Geometry check sheet. Reference: the model listing, model coordinates, mm. Face numbers are marked on the shaded views. A direction names the side the tool comes from. Round coordinates to 2 decimals unless told otherwise and drop trailing zeros. Order: outer loops, then holes, each group sorted by start corner. A loop starts at its lowest first (then second) coordinate and runs counter-clockwise, first axis right, second up.
(1) Cross-section at B-B on x = 26.5. Enter the section's corners in (y, z).
(2) Draft check along X on the marked faces 1, 2, 3 and 4. Enter one of: pulls with the +X half, pulls with the -X half, needs draft (parallel to the pull), parting line crosses it, or undercut.
(3) Gauge pin test, flat ends, axial feed: P1, Ø2, axis at x = 19.5, y = 10.5, coming from the +Z side; P2, Ø13.5, axis at y = 14.5, z = 5, coming from the +X side; P3, Ø3.5, axis at x = -6.5, z = 1.5, coming from the +Y side; P4, Ø11.5, axis at y = 25.5, z = 1, coming from the +X side. Record the tip position at first contact, or that the pin passes through.
(4) Cross-section at A-A on y = 25. Enter the section's corners in (x, z).
(5) Cross-section at D-D on y = 5. Enter the section's corners in (x, z), and give its area (4 significant figures).
(6) Thickness scan on L1, parallel to Z at x = 3.5, y = 7; L2, parallel to X at y = 8, z = 0; L3, parallel to Z at x = 23, y = 30.5. Record the ranges inside material, lowest first.
(7) Set-up check for the marked faces 5, 6 and 7: record each of +Z, -Z, +X, -X, +Y, -Y from which the full face is reachable in a straight line by a thin tool's end or side.
(8) Cross-section at C-C on z = 4.75. Enter the section's corners in (x, y), and give its area (3 significant figures).
from build123d import *

# Parameters (mm, degrees)
SKETCH1_W           = 38
SKETCH1_H           = 20
BOSS_EXTRUDE1_DEPTH = 32
SKETCH2_W           = 35
SKETCH2_H           = 17
CUT_EXTRUDE1_DEPTH  = 28
SKETCH3_W           = 4.5
SKETCH3_H           = 17
SKETCH3_W_2         = 6
BOSS_EXTRUDE2_DEPTH = 17.5
SKETCH4_W           = 44
SKETCH4_H           = 26
SKETCH4_W_2         = 38
SKETCH4_H_2         = 20
EXTRUDE_THIN2_DEPTH = 2


with BuildPart() as part:
    # Sketch1 → Boss-Extrude1 (new body)
    with BuildSketch(Plane(origin=(0, 0, 0), x_dir=(1, 0, 0), z_dir=(0, 1, 0))):
        with Locations((8.6, -4.057142857)):
            Rectangle(SKETCH1_W, SKETCH1_H)
    extrude(amount=BOSS_EXTRUDE1_DEPTH)

    # Sketch2 → Cut-Extrude1 (cut)
    with BuildSketch(Plane(origin=(0, 32, 0), x_dir=(1, 0, 0), z_dir=(0, 1, 0))):
        with Locations((8.5, -3.957142857)):
            Rectangle(SKETCH2_W, SKETCH2_H)
    extrude(amount=-CUT_EXTRUDE1_DEPTH, mode=Mode.SUBTRACT)

    # Sketch3 → Boss-Extrude2 (add)
    with BuildSketch(Plane(origin=(0, 4, 0), x_dir=(1, 0, 0), z_dir=(0, 1, 0))):
        with Locations((-6.75, -3.957142857)):
            Rectangle(SKETCH3_W, SKETCH3_H)
        with Locations((23, -3.957142857)):
            Rectangle(SKETCH3_W_2, SKETCH3_H)
    extrude(amount=BOSS_EXTRUDE2_DEPTH)

    # Sketch4 → Extrude-Thin2 (add)
    with BuildSketch(Plane(origin=(0, 32, 0), x_dir=(1, 0, 0), z_dir=(0, 1, 0))):
        with Locations((8.6, -4.057142857)):
            Rectangle(SKETCH4_W, SKETCH4_H)
        with Locations((8.6, -4.057142857)):
            Rectangle(SKETCH4_W_2, SKETCH4_H_2, mode=Mode.SUBTRACT)
    extrude(amount=-EXTRUDE_THIN2_DEPTH)


solid = part.part
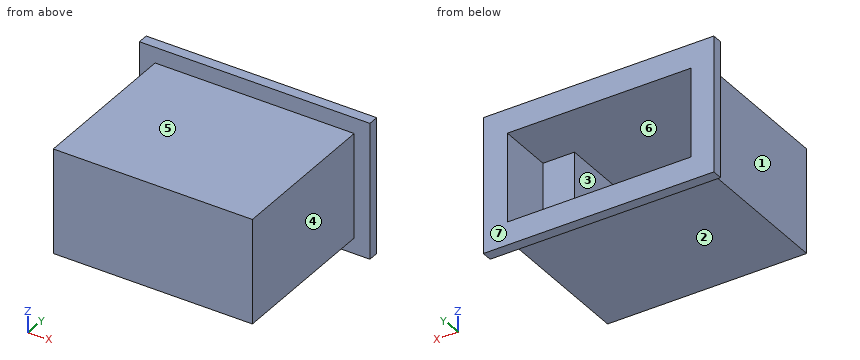
Found:
1. outline: (0, -5.94) - (30, -5.94) - (30, -8.94) - (32, -8.94) - (32, 17.06) - (30, 17.06) - (30, 14.06) - (0, 14.06) - close
2. face 1: pulls with the -X half
2. face 2: needs draft
2. face 3: undercut
2. face 4: pulls with the +X half
3. P1: stops at z = 14.06
3. P2: stops at x = 27.6
3. P3: stops at y = 21.5
3. P4: stops at x = 30.6
4. outline: (-10.4, -5.94) - (27.6, -5.94) - (27.6, 14.06) - (-10.4, 14.06) - close; hole (-9, -4.54) - (26, -4.54) - (26, 12.46) - (-9, 12.46) - close
5. outline: (-10.4, -5.94) - (27.6, -5.94) - (27.6, 14.06) - (-10.4, 14.06) - close; hole (-4.5, -4.54) - (20, -4.54) - (20, 12.46) - (-4.5, 12.46) - close
5. area: 343.5 mm2
6. L1: z = -5.94 to -4.54, 12.46 to 14.06
6. L2: x = -10.4 to -4.5, 20 to 27.6
6. L3: z = -8.94 to -4.54, 12.46 to 17.06
7. face 5: +Z, +X, -X, -Y
7. face 6: +Y
7. face 7: +Z, -Z, +X, -X, +Y
8. outline: (-13.4, 30) - (-10.4, 30) - (-10.4, 0) - (27.6, 0) - (27.6, 30) - (30.6, 30) - (30.6, 32) - (26, 32) - (26, 21.5) - (20, 21.5) - (20, 4) - (-4.5, 4) - (-4.5, 21.5) - (-9, 21.5) - (-9, 32) - (-13.4, 32) - close
8. area: 432 mm2
